```python
from build123d import *

# Parameters (mm, degrees)
HUB_FLANGE_PROFILE_R   = 30
HUB_FLANGE_PROFILE_R_2 = 3.25
HUB_FLANGE_5MM_DEPTH   = 5
STUB_AXLE_PROFILE_R    = 10
STUB_AXLE_75MM_DEPTH   = 75


with BuildPart() as part:
    # Hub_Flange_Profile → Hub_Flange_5mm (new body)
    with BuildSketch(Plane.XY):
        Circle(HUB_FLANGE_PROFILE_R)
        with Locations((20, 0)):
            Circle(HUB_FLANGE_PROFILE_R_2, mode=Mode.SUBTRACT)
        with Locations((0, 20)):
            Circle(HUB_FLANGE_PROFILE_R_2, mode=Mode.SUBTRACT)
        with Locations((-20, 0)):
            Circle(HUB_FLANGE_PROFILE_R_2, mode=Mode.SUBTRACT)
        with Locations((0, -20)):
            Circle(HUB_FLANGE_PROFILE_R_2, mode=Mode.SUBTRACT)
    extrude(amount=HUB_FLANGE_5MM_DEPTH)

    # Stub_Axle_Profile → Stub_Axle_75mm (add)
    with BuildSketch(Plane.XY):
        Circle(STUB_AXLE_PROFILE_R)
    extrude(amount=STUB_AXLE_75MM_DEPTH)


solid = part.part
```
Input: part model. Units: mm. Frame: model coordinates. A direction names the side the tool comes from. Coordinates: 2 decimals unless noted, no trailing zeros. Write each loop counter-clockwise with the first axis right and the second up, starting at its lowest first coordinate (ties: lowest second). Pieces come first, ordered by that corner, then holes. Notation, with made-up numbers: (28.25, 84) -> (66.25, 84) arc R7 ccw to (66.25, 92) -> close; hole circle Ø3 at (-32, 1.5). An arc over 180 degrees is marked (long way). Answer as a JSON object with one key per item and string values.
1. First-contact query: P1, Ø8, axis at x = -15, z = 9.5, coming from the -Y side; P2, Ø5, axis at x = -9, z = 59.5, coming from the -Y side; P3, Ø1, axis at y = -2, z = 59, coming from the +X side; P4, Ø10, axis at y = 12, z = 18.5, coming from the +X side. Flat tips, straight axial feed; report the tip coordinate or a pass-through.
Result set:
{"P1": "passes through", "P2": "stops at y = -7.6", "P3": "stops at x = 9.89", "P4": "stops at x = 7.14"}
2. Section D-D on x = -18.5. Return the cut outline in (y, z), then the cut area to 3 significant figures.
Result set:
{"outline": "(-23.62, 0) -> (-2.88, 0) -> (-2.88, 5) -> (-23.62, 5) -> close; (2.88, 0) -> (23.62, 0) -> (23.62, 5) -> (2.88, 5) -> close", "area": "207 mm2"}
3. Section A-A on y = 0. Return the cut outline in (x, z).
Result set:
{"outline": "(-30, 0) -> (-23.25, 0) -> (-23.25, 5) -> (-30, 5) -> close; (-16.75, 0) -> (16.75, 0) -> (16.75, 5) -> (10, 5) -> (10, 75) -> (-10, 75) -> (-10, 5) -> (-16.75, 5) -> close; (23.25, 0) -> (30, 0) -> (30, 5) -> (23.25, 5) -> close"}
4. Material intervals for line 1 (Y direction, x = 0, z = 4); line 2 (Z direction, x = 7.5, y = -9.5); line 3 (Y direction, x = -20, z = 2.7), sorted ascending. Write a range as from..to.
Result set:
{"line 1": "y = -30..-23.25, -16.75..16.75, 23.25..30", "line 2": "z = 0..5", "line 3": "y = -22.36..-3.25, 3.25..22.36"}
5. Access query for faces 1 (the face through (-0.423, -16.778, 2.465)), 2 (the face through (13, 0, 5)). Directions: +Z, -Z, +X, -X, +Y, -Y. A direction counts if a zero-diameter tool reaches every point of the face in a straight line with its end or side. Return the directions, or none.
Result set:
{"face 1": "+Z, -Z", "face 2": "+Z"}
6. Mould query, pull axis X, two halves, no side actions, for faces 3 (the face through (-29.97, 1.32, 2.46)), 4 (the face through (16.753, 0.143, 2.465)), 5 (the face through (0, 0, 0)). Classes: released by +X, released by -X, zero draft, split by the parting line, or undercut.
Result set:
{"face 3": "split by the parting line", "face 4": "undercut", "face 5": "zero draft"}
7. Section C-C on y = 19. Return the cut outline in (x, z).
Result set:
{"outline": "(-23.22, 0) -> (-3.09, 0) -> (-3.09, 5) -> (-23.22, 5) -> close; (3.09, 0) -> (23.22, 0) -> (23.22, 5) -> (3.09, 5) -> close"}
